The listing builds one solid part. Answer for the finished solid, in the listing's coordinates (mm). A direction names the side the tool comes from. Round coordinates to 2 decimals unless told otherwise and drop trailing zeros. Order: outer loops, then holes, each group sorted by start corner. A loop starts at its lowest first (then second) coordinate and runs counter-clockwise, first axis right, second up. Notation, with made-up numbers: M 54.5,-31.75 L 98.5,-31.75 A26 ccw 98.5,-7.75 Z; hole C 15,70 d1. An arc over 180 degrees is marked long. Put each result on its own line as item: value. Start each with the question number.
1. The part is cut by section C-C (x = 18). Give the vertices of the cut face in (y, z), then the cut area to 3 significant figures.
2. The part is cut by section A-A (y = -3). Give the vertices of the cut face in (x, z).
3. Each of these flat-tipped pins is pushed along its axis until it touches: pin 1 Ø2 at (x, y) = (1, 1.5) entering from -Z; pin 2 Ø1.5 at (x, z) = (20, 5.5) entering from +Y; pin 3 Ø3 at (y, z) = (11.5, 2.5) entering from -X; pin 4 Ø3 at (x, y) = (0, 0) entering from +Z. Where does it stop, or does it pass through?
4. The mould has two halves that part along Y. Classify faces 4 (the face through (-0.14, -12.09, 3.45)), 5 (the face through (-11.988, -1.571, 3.451)), 6 (the face through (2.664, 13.161, 3.451)): +Y half, -Y half, draft (parallel to the pull), parting line (faces both ways), or undercut.
5. Consider line 1 (X direction, y = 12.25, z = 2); line 2 (Y direction, x = 0, z = 5.75); line 3 (X direction, y = 13.5, z = 4.75). Determine where each line is inside the solid, lowest interval first.
6. Which of the six approach directions +Z, -Z, +X, -X, +Y, -Y give full straight-line access (tool end or side, diameter ignored) to faces 1 (the face through (-2.645, 13.128, 3.451)), 2 (the face through (11.996, 5.952, 3.451)), 3 (the face through (-7.422, 11.19, 3.451))?
7. The part is cut by section B-B (z = 6). Count the separate pieces of the cut face and the enclosed holes in it, then the cut area to 3 significant figures.
from build123d import *

# Parameters (mm, degrees)
SKETCH1_R           = 12.09
SKETCH1_R_2         = 1.75
BOSS_EXTRUDE2_DEPTH = 7
SKETCH2_R           = 3.5
CUT_EXTRUDE1_DEPTH  = 39.348395012
SKETCH3_R           = 3.5
SKETCH3_R_2         = 1.75
BOSS_EXTRUDE3_DEPTH = 2


with BuildPart() as part:
    # Sketch1 → Boss-Extrude2 (new body)
    # profile 1 of 17: a face of its own
    with BuildSketch(Plane.XY):
        Circle(SKETCH1_R)
    # profile 2 of 17: a face of its own
    with BuildSketch(Plane.XY):
        with BuildLine():
            ThreePointArc((-9.252623584, 7.781841479), (-8.548920985, 8.548920985), (-7.781841479, 9.252623584))
            ThreePointArc((-7.781841479, 9.252623584), (-8.870959341, 10.05645683), (-10.125769107, 10.564175311))
            Line((-10.125769107, 10.564175311), (-10.564175311, 10.125769107))
            ThreePointArc((-10.564175311, 10.125769107), (-10.05645683, 8.870959341), (-9.252623584, 7.781841479))
        make_face()
    # profile 3 of 17: a face of its own
    with BuildSketch(Plane.XY):
        with BuildLine():
            ThreePointArc((-6.9232593, 9.911436862), (-6.045, 10.470247132), (-5.12192646, 10.951436862))
            ThreePointArc((-5.12192646, 10.951436862), (-5.965886177, 12.009764599), (-7.046532125, 12.824951657))
            Line((-7.046532125, 12.824951657), (-7.583467875, 12.514951657))
            ThreePointArc((-7.583467875, 12.514951657), (-7.417818147, 11.171491285), (-6.9232593, 9.911436862))
        make_face()
    # profile 4 of 17: a face of its own
    with BuildSketch(Plane.XY):
        with BuildLine():
            ThreePointArc((-4.122086336, 11.365584201), (-3.129122255, 11.67804324), (-2.112960617, 11.903927815))
            ThreePointArc((-2.112960617, 11.903927815), (-2.65424773, 13.144626757), (-3.487085624, 14.211728743))
            Line((-3.487085624, 14.211728743), (-4.085959636, 14.051260935))
            ThreePointArc((-4.085959636, 14.051260935), (-4.273667417, 12.71070456), (-4.122086336, 11.365584201))
        make_face()
    # profile 5 of 17: a face of its own
    with BuildSketch(Plane.XY):
        with BuildLine():
            Line((0.31, 14.63), (-0.31, 14.63))
            ThreePointArc((-0.31, 14.63), (-0.838273314, 13.383704325), (-1.04, 12.04518576))
            ThreePointArc((-1.04, 12.04518576), (0, 12.09), (1.04, 12.04518576))
            ThreePointArc((1.04, 12.04518576), (0.838273314, 13.383704325), (0.31, 14.63))
        make_face()
    # profile 6 of 17: a face of its own
    with BuildSketch(Plane.XY):
        with BuildLine():
            ThreePointArc((3.487085624, 14.211728743), (2.65424773, 13.144626757), (2.112960617, 11.903927815))
            ThreePointArc((2.112960617, 11.903927815), (3.129122255, 11.67804324), (4.122086336, 11.365584201))
            ThreePointArc((4.122086336, 11.365584201), (4.273667417, 12.71070456), (4.085959636, 14.051260935))
            Line((4.085959636, 14.051260935), (3.487085624, 14.211728743))
        make_face()
    # profile 7 of 17: a face of its own
    with BuildSketch(Plane.XY):
        with BuildLine():
            ThreePointArc((7.046532125, 12.824951657), (5.965886177, 12.009764599), (5.12192646, 10.951436862))
            ThreePointArc((5.12192646, 10.951436862), (6.045, 10.470247132), (6.9232593, 9.911436862))
            ThreePointArc((6.9232593, 9.911436862), (7.417818147, 11.171491285), (7.583467875, 12.514951657))
            Line((7.583467875, 12.514951657), (7.046532125, 12.824951657))
        make_face()
    # profile 8 of 17: a face of its own
    with BuildSketch(Plane.XY):
        with BuildLine():
            ThreePointArc((10.125769107, 10.564175311), (8.870959341, 10.05645683), (7.781841479, 9.252623584))
            ThreePointArc((7.781841479, 9.252623584), (8.548920985, 8.548920985), (9.252623584, 7.781841479))
            ThreePointArc((9.252623584, 7.781841479), (10.05645683, 8.870959341), (10.564175311, 10.125769107))
            Line((10.564175311, 10.125769107), (10.125769107, 10.564175311))
        make_face()
    # profile 9 of 17: a face of its own
    with BuildSketch(Plane.XY):
        with BuildLine():
            ThreePointArc((12.514951657, 7.583467875), (11.171491285, 7.417818147), (9.911436862, 6.9232593))
            ThreePointArc((9.911436862, 6.9232593), (10.470247132, 6.045), (10.951436862, 5.12192646))
            ThreePointArc((10.951436862, 5.12192646), (12.009764599, 5.965886177), (12.824951657, 7.046532125))
            Line((12.824951657, 7.046532125), (12.514951657, 7.583467875))
        make_face()
    # profile 10 of 17: a face of its own
    with BuildSketch(Plane.XY):
        with BuildLine():
            Line((14.07429375, 4), (11.409123542, 4))
            ThreePointArc((11.409123542, 4), (11.694649217, 3.066476756), (11.903927815, 2.112960617))
            ThreePointArc((11.903927815, 2.112960617), (13.144626757, 2.65424773), (14.211728743, 3.487085624))
            Line((14.211728743, 3.487085624), (14.07429375, 4))
        make_face()
    # profile 11 of 17: a face of its own
    with BuildSketch(Plane.XY):
        with BuildLine():
            Line((30.75, 4), (14.07429375, 4))
            Line((14.07429375, 4), (14.211728743, 3.487085624))
            ThreePointArc((14.211728743, 3.487085624), (13.144626757, 2.65424773), (11.903927815, 2.112960617))
            ThreePointArc((11.903927815, 2.112960617), (11.986568374, 1.578061664), (12.04518576, 1.04))
            ThreePointArc((12.04518576, 1.04), (13.383704325, 0.838273314), (14.63, 0.31))
            Line((14.63, 0.31), (14.63, -0.31))
            ThreePointArc((14.63, -0.31), (13.383704325, -0.838273314), (12.04518576, -1.04))
            ThreePointArc((12.04518576, -1.04), (11.986568374, -1.578061664), (11.903927815, -2.112960617))
            ThreePointArc((11.903927815, -2.112960617), (13.144626757, -2.65424773), (14.211728743, -3.487085624))
            Line((14.211728743, -3.487085624), (14.07429375, -4))
            Line((14.07429375, -4), (30.75, -4))
            ThreePointArc((30.75, -4), (34.75, 0), (30.75, 4))
        make_face()
        with Locations((30.75, 0)):
            Circle(SKETCH1_R_2, mode=Mode.SUBTRACT)
    # profile 12 of 17: a face of its own
    with BuildSketch(Plane.XY):
        with BuildLine():
            ThreePointArc((14.63, 0.31), (13.383704325, 0.838273314), (12.04518576, 1.04))
            ThreePointArc((12.04518576, 1.04), (12.078791244, 0.520482544), (12.09, 0))
            ThreePointArc((12.09, 0), (12.078791244, -0.520482544), (12.04518576, -1.04))
            ThreePointArc((12.04518576, -1.04), (13.383704325, -0.838273314), (14.63, -0.31))
            Line((14.63, -0.31), (14.63, 0.31))
        make_face()
    # profile 13 of 17: a face of its own
    with BuildSketch(Plane.XY):
        with BuildLine():
            Line((11.409123542, -4), (14.07429375, -4))
            Line((14.07429375, -4), (14.211728743, -3.487085624))
            ThreePointArc((14.211728743, -3.487085624), (13.144626757, -2.65424773), (11.903927815, -2.112960617))
            ThreePointArc((11.903927815, -2.112960617), (11.694649217, -3.066476756), (11.409123542, -4))
        make_face()
    # profile 14 of 17: a face of its own
    with BuildSketch(Plane.XY):
        with BuildLine():
            ThreePointArc((-10.951436862, 5.12192646), (-10.470247132, 6.045), (-9.911436862, 6.9232593))
            ThreePointArc((-9.911436862, 6.9232593), (-11.171491285, 7.417818147), (-12.514951657, 7.583467875))
            Line((-12.514951657, 7.583467875), (-12.824951657, 7.046532125))
            ThreePointArc((-12.824951657, 7.046532125), (-12.009764599, 5.965886177), (-10.951436862, 5.12192646))
        make_face()
    # profile 15 of 17: a face of its own
    with BuildSketch(Plane.XY):
        with BuildLine():
            ThreePointArc((-11.903927815, 2.112960617), (-11.67804324, 3.129122255), (-11.365584201, 4.122086336))
            ThreePointArc((-11.365584201, 4.122086336), (-12.71070456, 4.273667417), (-14.051260935, 4.085959636))
            Line((-14.051260935, 4.085959636), (-14.211728743, 3.487085624))
            ThreePointArc((-14.211728743, 3.487085624), (-13.144626757, 2.65424773), (-11.903927815, 2.112960617))
        make_face()
    # profile 16 of 17: a face of its own
    with BuildSketch(Plane.XY):
        with BuildLine():
            ThreePointArc((-12.04518576, -1.04), (-12.09, 0), (-12.04518576, 1.04))
            ThreePointArc((-12.04518576, 1.04), (-13.383704325, 0.838273314), (-14.63, 0.31))
            Line((-14.63, 0.31), (-14.63, -0.31))
            ThreePointArc((-14.63, -0.31), (-13.383704325, -0.838273314), (-12.04518576, -1.04))
        make_face()
    # profile 17 of 17: a face of its own
    with BuildSketch(Plane.XY):
        with BuildLine():
            ThreePointArc((-11.365584201, -4.122086336), (-11.67804324, -3.129122255), (-11.903927815, -2.112960617))
            ThreePointArc((-11.903927815, -2.112960617), (-13.144626757, -2.65424773), (-14.211728743, -3.487085624))
            Line((-14.211728743, -3.487085624), (-14.051260935, -4.085959636))
            ThreePointArc((-14.051260935, -4.085959636), (-12.71070456, -4.273667417), (-11.365584201, -4.122086336))
        make_face()
    extrude(amount=BOSS_EXTRUDE2_DEPTH)

    # Sketch2 → Cut-Extrude1 (cut, through all)
    with BuildSketch(Plane.XY.offset(7)):
        Circle(SKETCH2_R)
    extrude(amount=-CUT_EXTRUDE1_DEPTH, mode=Mode.SUBTRACT)

    # Sketch3 → Boss-Extrude3 (add)
    with BuildSketch(Plane.XY.offset(7)):
        Circle(SKETCH3_R)
        Circle(SKETCH3_R_2, mode=Mode.SUBTRACT)
    extrude(amount=-BOSS_EXTRUDE3_DEPTH)


solid = part.part
Resolved:
1. outline: M -4,0 L 4,0 L 4,7 L -4,7 Z
1. area: 56.0 mm2
2. outline: M -13.66,0 L -1.8,0 L -1.8,5 L 1.8,5 L 1.8,0 L 33.4,0 L 33.4,7 L -13.66,7 Z
3. pin 1: z = 5
3. pin 2: y = 4
3. pin 3: x = -10.56
3. pin 4: through
4. face 4: -Y half
4. face 5: undercut
4. face 6: +Y half
5. line 1: -7.58 to -6.23, -4.26 to -2.23, -1.03 to 1.03, 2.23 to 4.26, 6.23 to 7.58
5. line 2: -12.09 to -1.75, 1.75 to 14.63
5. line 3: -4.2 to -2.89, -0.8 to 0.8, 2.89 to 4.2
6. face 1: +Z, -Z, +Y
6. face 2: +Z, -Z, +X
6. face 3: +Z, -Z
7. separate pieces: 1
7. enclosed holes: 2
7. area: 665 mm2
